Source: CAD feature listing. Evaluate the final solid. Frame: model axes, mm. A direction names the side the tool comes from. Give positions to 0.01 mm unless a question says otherwise; leave off trailing zeros. Order: outer loops, then holes, each group sorted by start corner. A loop starts at its lowest first (then second) coordinate and runs counter-clockwise, first axis right, second up. Notation, with made-up numbers: M 23.5,19 L 76.5,19 A29 cw 76.5,53 Z; hole C 76.25,6 d7. An arc over 180 degrees is marked long. Answer as a JSON object with one key per item and string values. Group by question number.
1. Section query D-D (y = 12.5). Output: boundary loops of the cut face in (x, z).
2. Pin query (flat end, axial travel): P1, Ø0.9, axis at y = 25, z = 6.5, coming from the +X side; P2, Ø1.5, axis at x = -87.5, z = 2.5, coming from the +Y side; P3, Ø1.5, axis at x = -89, z = 3, coming from the -Y side; P4, Ø2.5, axis at y = 45.5, z = 6, coming from the -X side. Return the tip coordinate at first contact, or that it passes through.
3. Material intervals for L1, parallel to Y at x = -4.5, z = 3.6; L2, parallel to Y at x = -88, z = 1; L3, parallel to X at y = 42.5, z = 2.5, sorted ascending. Write a range as [from, to].
4. Section query B-B (z = 6.5). Output: boundary loops of the cut face in (x, y).
5. Section query C-C (x = -49.5). Output: boundary loops of the cut face in (y, z), plus the area to 4 significant figures.
6. Section query A-A (y = 30). Output: boundary loops of the cut face in (x, z), plus the area to 3 significant figures.
7. Set-up query: faces 4 (the flat face through (-43, 0, 2)), 5 (the flat face through (-83, 72, 2)), 6 (the flat face through (-52, 53.85, 3)), 7 (the flat face through (-21.96, 3.22, 8.13)), 8 (the flat face through (-14, 24, 8)). Return all of +Z, -Z, +X, -X, +Y, -Y with unobstructed straight access to the full face (end or side cutting, diameter ignored); none if empty.
8. Pull-direction query (X, two-part tool) for faces 1 (the flat face through (-78, 2, 2)), 2 (the flat face through (-97, 33, 2)), 3 (the flat face through (-10, 0, 2)); classes: +X half, -X half, draft (parallel to the pull), parting line (faces both ways), or undercut.
from build123d import *

# Parameters (mm, degrees)
SKETCH1_W           = 97
SKETCH1_H           = 67.7
BOSS_EXTRUDE1_DEPTH = 5
SKETCH2_R           = 2
SKETCH2_R_2         = 1.5
SKETCH2_W           = 60
SKETCH2_H           = 40
CUT_EXTRUDE1_DEPTH  = 6
SKETCH3_W           = 3
SKETCH3_H           = 5
SKETCH3_W_2         = 5
SKETCH3_H_2         = 7
BOSS_EXTRUDE2_DEPTH = 3
SKETCH7_W           = 5
SKETCH7_H           = 11.35
BOSS_EXTRUDE4_DEPTH = 30
BOSS_EXTRUDE5_DEPTH = 5
SKETCH4_W           = 12.75
SKETCH4_H           = 12.75
CUT_EXTRUDE2_DEPTH  = 12.35
BOSS_EXTRUDE6_DEPTH = 5


with BuildPart() as part:
    # Sketch1 → Boss-Extrude1 (new body)
    with BuildSketch(Plane.XY):
        with Locations((-48.5, 33.85)):
            Rectangle(SKETCH1_W, SKETCH1_H)
    extrude(amount=BOSS_EXTRUDE1_DEPTH)

    # Sketch2 → Cut-Extrude1 (cut, through all)
    with BuildSketch(Plane.XY.offset(5)):
        with Locations((-88, 34.2)):
            Circle(SKETCH2_R)
        with Locations((-4.5, 49.2)):
            Circle(SKETCH2_R_2)
        with Locations((-52, 33.85)):
            Rectangle(SKETCH2_W, SKETCH2_H)
    extrude(amount=-CUT_EXTRUDE1_DEPTH, mode=Mode.SUBTRACT)

    # Sketch3 → Boss-Extrude2 (add)
    with BuildSketch(Plane.XY.offset(5)):
        with Locations((-90.5, 44.7)):
            Rectangle(SKETCH3_W, SKETCH3_H)
        with Locations((-90.5, 23.7)):
            Rectangle(SKETCH3_W, SKETCH3_H)
        with Locations((-14, 45.45)):
            Rectangle(SKETCH3_W_2, SKETCH3_H_2)
        with Locations((-14, 24.45)):
            Rectangle(SKETCH3_W_2, SKETCH3_H_2)
    extrude(amount=BOSS_EXTRUDE2_DEPTH)

    # Sketch7 → Boss-Extrude4 (add)
    with BuildSketch(Plane.XZ):
        with Locations((-22, 5.675)):
            Rectangle(SKETCH7_W, SKETCH7_H)
    extrude(amount=BOSS_EXTRUDE4_DEPTH)

    # Sketch8 → Boss-Extrude5 (add)
    with BuildSketch(Plane(origin=(-19.5, 0, 0), x_dir=(0, 0, -1), z_dir=(1, 0, 0))):
        Polygon((-11.35, 0), (-5, 0), (-5, 6.35), align=None)
    extrude(amount=-BOSS_EXTRUDE5_DEPTH)

    # Sketch4 → Cut-Extrude2 (cut, through all)
    with BuildSketch(Plane(origin=(0, 0, 0), x_dir=(-1, 0, 0), z_dir=(0, 0, -1))):
        with Locations((71.625, 65.225)):
            Rectangle(SKETCH4_W, SKETCH4_H)
        with Locations((71.625, 2.475)):
            Rectangle(SKETCH4_W, SKETCH4_H)
    extrude(amount=-CUT_EXTRUDE2_DEPTH, mode=Mode.SUBTRACT)

    # Sketch10 → Boss-Extrude6 (add)
    with BuildSketch(Plane(origin=(0, 0, 0), x_dir=(-1, 0, 0), z_dir=(0, 0, -1))):
        Polygon((83, 0), (83, -8.9), (60.25, -8.9), (60.25, 0), (65.25, 0), (65.25, -3.9), (78, -3.9), (78, 0), align=None)
        Polygon((83, 67.7), (78, 67.7), (78, 71.6), (65.25, 71.6), (65.25, 67.7), (60.25, 67.7), (60.25, 76.6), (83, 76.6), align=None)
    extrude(amount=-BOSS_EXTRUDE6_DEPTH)


solid = part.part
Answer sheet:
{
 "1": {"outline": "M -97,0 L 0,0 L 0,5 L -97,5 Z"},
 "2": {"P1": "x = -11.5", "P2": "y = 67.7", "P3": "y = 0", "P4": "x = -97"},
 "3": {"L1": "[0, 47.7], [50.7, 67.7]", "L2": "[0, 32.2], [36.2, 67.7]", "L3": "[-97, -82], [-22, 0]"},
 "4": {"outline": "M -92,21.2 L -89,21.2 L -89,26.2 L -92,26.2 Z; M -92,42.2 L -89,42.2 L -89,47.2 L -92,47.2 Z; M -24.5,-30 L -19.5,-30 L -19.5,4.85 L -24.5,4.85 Z; M -16.5,20.95 L -11.5,20.95 L -11.5,27.95 L -16.5,27.95 Z; M -16.5,41.95 L -11.5,41.95 L -11.5,48.95 L -16.5,48.95 Z"},
 "5": {"outline": "M 0,0 L 13.85,0 L 13.85,5 L 0,5 Z; M 53.85,0 L 67.7,0 L 67.7,5 L 53.85,5 Z", "area": "138.5 mm^2"},
 "6": {"outline": "M -97,0 L -82,0 L -82,5 L -97,5 Z; M -22,0 L 0,0 L 0,5 L -22,5 Z", "area": "185 mm^2"},
 "7": {"face 4": "+Z, -Z, -Y", "face 5": "+Z, -Z, -X, +Y", "face 6": "+Z, -Z", "face 7": "+Z, +X, -X, +Y", "face 8": "+Z, +X, -X, +Y, -Y"},
 "8": {"face 1": "undercut", "face 2": "-X half", "face 3": "draft"}
}
